```python
from build123d import *

# Parameters (mm, degrees)
F0_W     = 30
F0_H     = 50
F1_DEPTH = 10
F2_SIZE  = 4.99999


# Not quite as in the source:
# - a fillet or chamfer is up to 0.001 mm smaller than in the source, because OpenCascade refuses the exact size


with BuildPart() as f1:
    # F0 (on Right) → F1 (new body)
    with BuildSketch(Plane.YZ):
        Rectangle(F0_W, F0_H)
    extrude(amount=F1_DEPTH)

    # F2 (size 5 in the source; OpenCascade refuses exactly that, so slightly less here)
    f2_edges = [f1.edges().sort_by_distance(p)[0] for p in [
        (5, -15, 25),
        (5, -15, -25),
        (0, -15, 0),
        (10, -15, 0),
        (5, 15, -25),
        (5, 15, 25),
        (0, 15, 0),
        (10, 15, 0),
        (10, 0, 25),
        (10, 0, -25),
        (0, 0, 25),
        (0, 0, -25),
    ]]
    chamfer(f2_edges, length=F2_SIZE)


solid = f1.part
```
The listing builds one solid part. Answer for the finished solid, in the listing's coordinates (mm). Give positions to 0.01 mm unless a question says otherwise; leave off trailing zeros. One line per item, written item: value.
1. For a pull along Y with two mould halves and no side action, classify faces 1 (the face through (2, 12, 0)), 2 (the face through (6.9, -11.6, -21.5)), 3 (the face through (2, 0, 22)) as pulls with the +Y half, pulls with the -Y half, needs draft (parallel to the pull), parting line crosses it, or undercut.
Found:
face 1: pulls with the +Y half
face 2: pulls with the -Y half
face 3: needs draft
2. Each of these flat-tipped pins is pushed along its axis until it touches: P1, Ø6, axis at x = 4, z = -16, coming from the +Y side; P2, Ø3, axis at x = 4.5, y = 7, coming from the -Z side; P3, Ø2, axis at x = 2.5, z = 0, coming from the +Y side. Where does it stop, or does it pass through?
Found:
P1: y = 15
P2: z = -25
P3: y = 13.5
3. Find the intervals of material crossed by probe 1 along Y at (x, z) = (4, 8); probe 2 along Z at (x, y) = (5.75, -6.5); probe 3 along X at (y, z) = (14, -18), in increasing order.
Found:
probe 1: -14 to 14
probe 2: -24.25 to 24.25
probe 3: 4 to 6
